Answer from the drawing. Dimensions are ordinates in mm from the lowest x, y and z of the part. A direction names the side the tool comes from. Give positions to 0.01 mm unless a question says otherwise; leave off trailing zeros. Write each loop counter-clockwise with the first axis right and the second up, starting at its lowest first coordinate (ties: lowest second). Pieces come first, ordered by that corner, then holes. Notation, with made-up numbers: (88.25, -7.5) -> (96.25, -7.5) arc R26 ccw to (96.25, 25.5) -> close; hole circle Ø10 at (77.25, 77.5). An arc over 180 degrees is marked (long way). Put each result on its own line as item: value. Start each with the question number.
1) A cutting plane is placed at B-B (z = 4.75). Write down the section's boundary in (x, y), then the cut area to 3 significant figures.
2) For a pull along X with two mould halves and no side action, classify the marked faces 3, 4, 5 and 6 as released by +X, released by -X, zero draft, split by the parting line, or undercut.
3) Find the intervals of material crossed by line 1 along Y through (x, z) = (9.5, 4.25); line 2 along X through (y, z) = (21, 6); line 3 along X through (y, z) = (9, 2.5), in increasing order. Write a range as from..to.
4) A cutting plane is placed at C-C (x = 40.5). Write down the section's boundary in (y, z), then the cut area to 3 significant figures.
5) A cutting plane is placed at D-D (y = 36.5). Write down the section's boundary in (x, z).
6) A cutting plane is placed at A-A (y = 11). Write down the section's boundary in (x, z).
7) For the marked faces 1 and 2, determine the directions among +Z, -Z, +X, -X, +Y, -Y from which every point of the face is accessible in a straight line to the end or side of a thin tool.
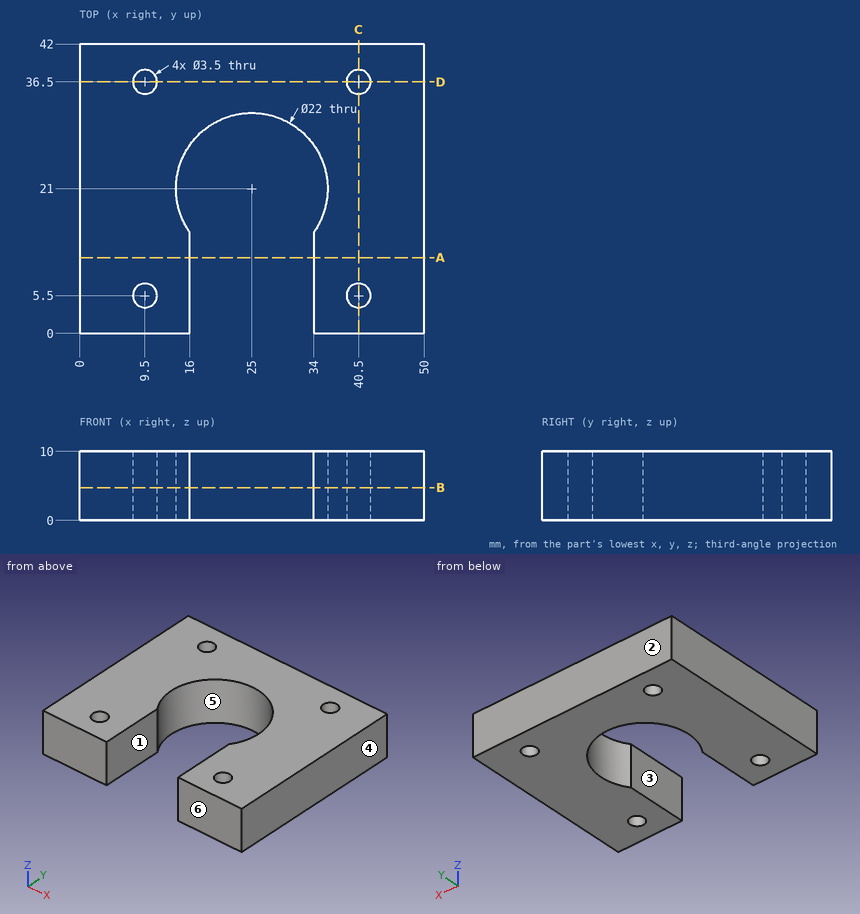
Reply:
1. outline: (0, 0) -> (16, 0) -> (16, 14.68) arc R11 cw (long way) to (34, 14.68) -> (34, 0) -> (50, 0) -> (50, 42) -> (0, 42) -> close; hole circle Ø3.5 at (9.5, 5.5); hole circle Ø3.5 at (9.5, 36.5); hole circle Ø3.5 at (40.5, 5.5); hole circle Ø3.5 at (40.5, 36.5)
1. area: 1,480 mm2
2. face 3: undercut
2. face 4: released by +X
2. face 5: undercut
2. face 6: zero draft
3. line 1: y = 0..3.75, 7.25..34.75, 38.25..42
3. line 2: x = 0..14, 36..50
3. line 3: x = 0..16, 34..50
4. outline: (0, 0) -> (3.75, 0) -> (3.75, 10) -> (0, 10) -> close; (7.25, 0) -> (34.75, 0) -> (34.75, 10) -> (7.25, 10) -> close; (38.25, 0) -> (42, 0) -> (42, 10) -> (38.25, 10) -> close
4. area: 350 mm2
5. outline: (0, 0) -> (7.75, 0) -> (7.75, 10) -> (0, 10) -> close; (11.25, 0) -> (38.75, 0) -> (38.75, 10) -> (11.25, 10) -> close; (42.25, 0) -> (50, 0) -> (50, 10) -> (42.25, 10) -> close
6. outline: (0, 0) -> (16, 0) -> (16, 10) -> (0, 10) -> close; (34, 0) -> (50, 0) -> (50, 10) -> (34, 10) -> close
7. face 1: +Z, -Z, -Y
7. face 2: +Z, -Z, +X, -X, +Y
